Part model, mm, in its own coordinate system. Give positions to 0.01 mm unless a question says otherwise; leave off trailing zeros. Use a Markdown table: item, result. Add a question column.
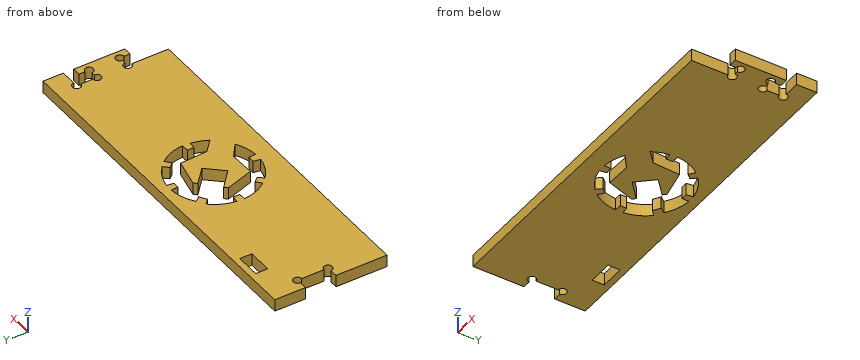
from build123d import *

# Parameters (mm, degrees)
SKETCH1_W           = 164.9
SKETCH1_H           = 55
BOSS_EXTRUDE1_DEPTH = 5.9
SKETCH2_W           = 5.9
SKETCH2_H           = 15
CUT_EXTRUDE1_DEPTH  = 6.9
BOSS_EXTRUDE2_DEPTH = 5.9
CUT_EXTRUDE2_DEPTH  = 10
SKETCH5_W           = 10
SKETCH5_H           = 10
BOSS_EXTRUDE3_DEPTH = 5.9
CUT_EXTRUDE3_REACH  = 7.9
SKETCH6_R           = 2.05
CUT_EXTRUDE4_REACH  = 7.9
SKETCH7_W           = 12
SKETCH7_H           = 5.9


with BuildPart() as part:
    # Sketch1 → Boss-Extrude1 (new body)
    with BuildSketch(Plane.XY):
        Rectangle(SKETCH1_W, SKETCH1_H)
    extrude(amount=BOSS_EXTRUDE1_DEPTH)

    # Sketch2 → Cut-Extrude1 (cut, through all)
    with BuildSketch(Plane.XY.offset(5.9)):
        with Locations((-79.5, 5)):
            Rectangle(SKETCH2_W, SKETCH2_H)
    extrude(amount=-CUT_EXTRUDE1_DEPTH, mode=Mode.SUBTRACT)

    # Sketch3 → Boss-Extrude2 (add)
    with BuildSketch(Plane.XY.offset(5.9)):
        Polygon((82.45, -7.5), (88.35, -7.5), (88.35, -12.5), (92.35, -12.5), (92.35, 12.5), (88.35, 12.5), (88.35, 7.5), (82.45, 7.5), align=None)
    extrude(amount=-BOSS_EXTRUDE2_DEPTH)

    # Sketch4 → Cut-Extrude2 (cut)
    with BuildSketch(Plane.XY.offset(5.9)):
        with BuildLine():
            Line((3.51583171, -15.706229716), (3.692822505, -19.080784973))
            ThreePointArc((3.692822505, -19.080784973), (9.080825588, -18.035079597), (14.033003188, -15.668644733))
            Line((14.033003188, -15.668644733), (7.525249631, -10.707966449))
            Line((7.525249631, -10.707966449), (-4.667323255, -11.041732232))
            Line((-4.667323255, -11.041732232), (-9.056316648, 2.465721032))
            Line((-9.056316648, 2.465721032), (-7.672540361, 3.987452797))
            Line((-7.672540361, 3.987452797), (0.63828327, -3.480150804))
            Line((0.63828327, -3.480150804), (7.889093057, 4.589420993))
            Line((7.889093057, 4.589420993), (0.219729645, 11.480963368))
            Line((0.219729645, 11.480963368), (1.603052795, 13.017301391))
            Line((1.603052795, 13.017301391), (15.495445969, 10.065059871))
            Line((15.495445969, 10.065059871), (16.237659976, -3.337384453))
            Line((16.237659976, -3.337384453), (21.895941701, -8.451220184))
            ThreePointArc((21.895941701, -8.451220184), (23.579573726, -4.648525456), (24.507536721, -0.594639829))
            Line((24.507536721, -0.594639829), (21.171770806, -0.180639971))
            ThreePointArc((21.171770806, -0.180639971), (21.286498935, 1.378538101), (21.285888417, 2.941931343))
            Line((21.285888417, 2.941931343), (24.837258291, 3.128195824))
            ThreePointArc((24.837258291, 3.128195824), (23.536690781, 9.458573353), (20.269548114, 15.034497878))
            Line((20.269548114, 15.034497878), (17.535016414, 12.941488009))
            ThreePointArc((17.535016414, 12.941488009), (16.508769514, 14.081533134), (15.445096221, 15.186741129))
            Line((15.445096221, 15.186741129), (17.692052457, 17.680150482))
            ThreePointArc((17.692052457, 17.680150482), (12.304554027, 21.210935864), (6.104308905, 22.956944215))
            Line((6.104308905, 22.956944215), (5.70284553, 19.6211861))
            ThreePointArc((5.70284553, 19.6211861), (4.176993745, 19.749298528), (2.645876068, 19.73154678))
            Line((2.645876068, 19.73154678), (2.474568352, 23.105152619))
            ThreePointArc((2.474568352, 23.105152619), (-3.819532601, 21.764454936), (-9.443176471, 18.635907879))
            Line((-9.443176471, 18.635907879), (-7.36611055, 15.97938168))
            ThreePointArc((-7.36611055, 15.97938168), (-9.138032671, 15.057329352), (-10.764172697, 13.897347837))
            Line((-10.764172697, 13.897347837), (-13.255215364, 16.14691078))
            ThreePointArc((-13.255215364, 16.14691078), (-16.804652941, 10.7695067), (-18.541993583, 4.564941506))
            Line((-18.541993583, 4.564941506), (-15.203305308, 4.160483172))
            ThreePointArc((-15.203305308, 4.160483172), (-15.337848427, 2.624728095), (-15.310082988, 1.083340867))
            Line((-15.310082988, 1.083340867), (-18.663730537, 0.907446652))
            ThreePointArc((-18.663730537, 0.907446652), (-17.372056658, -5.384049821), (-14.221680713, -10.981056224))
            Line((-14.221680713, -10.981056224), (-11.574159014, -8.917273625))
            ThreePointArc((-11.574159014, -8.917273625), (-10.549530454, -10.048759249), (-9.495391581, -11.15280392))
            Line((-9.495391581, -11.15280392), (-11.74257315, -13.641863724))
            ThreePointArc((-11.74257315, -13.641863724), (-6.357210629, -17.182483384), (-0.156549988, -18.940301546))
            Line((-0.156549988, -18.940301546), (0.271448667, -15.602569205))
            ThreePointArc((0.271448667, -15.602569205), (1.891578011, -15.718941802), (3.51583171, -15.706229716))
        make_face()
    extrude(amount=-CUT_EXTRUDE2_DEPTH, mode=Mode.SUBTRACT)

    # Sketch5 → Boss-Extrude3 (add)
    with BuildSketch(Plane(origin=(0, 0, 0), x_dir=(-1, 0, 0), z_dir=(0, 0, -1))):
        with Locations((-87.45, 22.5)):
            Rectangle(SKETCH5_W, SKETCH5_H)
    extrude(amount=-BOSS_EXTRUDE3_DEPTH)

    # Sketch6 → Cut-Extrude3 (cut, up to next)
    with BuildSketch(Plane(origin=(0, 0, 0), x_dir=(-1, 0, 0), z_dir=(0, 0, -1)), mode=Mode.PRIVATE) as cut_extrude3_sk1:
        with Locations((-82.45, -7.5)):
            Circle(SKETCH6_R)
    cut_extrude3_tool1 = extrude(cut_extrude3_sk1.sketch, amount=-CUT_EXTRUDE3_REACH, mode=Mode.PRIVATE) & part.part
    add(cut_extrude3_tool1.solids().sort_by_distance((82.45, -7.5, 0))[0], mode=Mode.SUBTRACT)
    # Sketch6 → Cut-Extrude3 (cut, up to next)
    with BuildSketch(Plane(origin=(0, 0, 0), x_dir=(-1, 0, 0), z_dir=(0, 0, -1)), mode=Mode.PRIVATE) as cut_extrude3_sk2:
        with Locations((-88.35, -7.5)):
            Circle(SKETCH6_R)
    cut_extrude3_tool2 = extrude(cut_extrude3_sk2.sketch, amount=-CUT_EXTRUDE3_REACH, mode=Mode.PRIVATE) & part.part
    add(cut_extrude3_tool2.solids().sort_by_distance((88.35, -7.5, 0))[0], mode=Mode.SUBTRACT)
    # Sketch6 → Cut-Extrude3 (cut, up to next)
    with BuildSketch(Plane(origin=(0, 0, 0), x_dir=(-1, 0, 0), z_dir=(0, 0, -1)), mode=Mode.PRIVATE) as cut_extrude3_sk3:
        with Locations((-88.35, 7.5)):
            Circle(SKETCH6_R)
    cut_extrude3_tool3 = extrude(cut_extrude3_sk3.sketch, amount=-CUT_EXTRUDE3_REACH, mode=Mode.PRIVATE) & part.part
    add(cut_extrude3_tool3.solids().sort_by_distance((88.35, 7.5, 0))[0], mode=Mode.SUBTRACT)
    # Sketch6 → Cut-Extrude3 (cut, up to next)
    with BuildSketch(Plane(origin=(0, 0, 0), x_dir=(-1, 0, 0), z_dir=(0, 0, -1)), mode=Mode.PRIVATE) as cut_extrude3_sk4:
        with Locations((-82.45, 7.5)):
            Circle(SKETCH6_R)
    cut_extrude3_tool4 = extrude(cut_extrude3_sk4.sketch, amount=-CUT_EXTRUDE3_REACH, mode=Mode.PRIVATE) & part.part
    add(cut_extrude3_tool4.solids().sort_by_distance((82.45, 7.5, 0))[0], mode=Mode.SUBTRACT)
    # Sketch6 → Cut-Extrude3 (cut, up to next)
    with BuildSketch(Plane(origin=(0, 0, 0), x_dir=(-1, 0, 0), z_dir=(0, 0, -1)), mode=Mode.PRIVATE) as cut_extrude3_sk5:
        with Locations((-82.45, 17.5)):
            Circle(SKETCH6_R)
    cut_extrude3_tool5 = extrude(cut_extrude3_sk5.sketch, amount=-CUT_EXTRUDE3_REACH, mode=Mode.PRIVATE) & part.part
    add(cut_extrude3_tool5.solids().sort_by_distance((82.45, 17.5, 0))[0], mode=Mode.SUBTRACT)
    # Sketch6 → Cut-Extrude3 (cut, up to next)
    with BuildSketch(Plane(origin=(0, 0, 0), x_dir=(-1, 0, 0), z_dir=(0, 0, -1)), mode=Mode.PRIVATE) as cut_extrude3_sk6:
        with Locations((76.55, 12.5)):
            Circle(SKETCH6_R)
    cut_extrude3_tool6 = extrude(cut_extrude3_sk6.sketch, amount=-CUT_EXTRUDE3_REACH, mode=Mode.PRIVATE) & part.part
    add(cut_extrude3_tool6.solids().sort_by_distance((-76.55, 12.5, 0))[0], mode=Mode.SUBTRACT)
    # Sketch6 → Cut-Extrude3 (cut, up to next)
    with BuildSketch(Plane(origin=(0, 0, 0), x_dir=(-1, 0, 0), z_dir=(0, 0, -1)), mode=Mode.PRIVATE) as cut_extrude3_sk7:
        with Locations((76.55, -2.5)):
            Circle(SKETCH6_R)
    cut_extrude3_tool7 = extrude(cut_extrude3_sk7.sketch, amount=-CUT_EXTRUDE3_REACH, mode=Mode.PRIVATE) & part.part
    add(cut_extrude3_tool7.solids().sort_by_distance((-76.55, -2.5, 0))[0], mode=Mode.SUBTRACT)

    # Sketch7 → Cut-Extrude4 (cut, up to next)
    with BuildSketch(Plane(origin=(0, 0, 0), x_dir=(-1, 0, 0), z_dir=(0, 0, -1)), mode=Mode.PRIVATE) as cut_extrude4_sk1:
        with Locations((57.45, 21.55)):
            Rectangle(SKETCH7_W, SKETCH7_H)
    cut_extrude4_tool1 = extrude(cut_extrude4_sk1.sketch, amount=-CUT_EXTRUDE4_REACH, mode=Mode.PRIVATE) & part.part
    add(cut_extrude4_tool1.solids().sort_by_distance((-57.45, 21.55, 0))[0], mode=Mode.SUBTRACT)


solid = part.part
1. Cut at A-A (z = 2). State how many separate pieces and enclosed holes the cut face has, plus the area to 3 significant figures.
2. Drill centre lines: probe 1 along Y at (x, z) = (-3, 3.2); probe 2 along X at (y, z) = (13.5, 1.15); probe 3 along X at (y, z) = (-14.5, 4.95). Where is each one in solid material? Low to high. Write a range as [from, to].
3. Pin check, flat tips, straight feed: P1, Ø8, axis at x = 11, y = 15, coming from the -Z side; P2, Ø2.5, axis at x = 82.45, y = -7.5, coming from the +Z side; P3, Ø1, axis at y = 5, z = 3.5, coming from the -X side; P4, Ø3, axis at y = 2.5, z = 4, coming from the +X side. Stop position of each tip, or through.
Responses:
| question | item | result |
|---|---|---|
| 1 | separate pieces | 1 |
| 1 | enclosed holes | 2 |
| 1 | area | 8,210 mm² |
| 2 | probe 1 | y = [-27.5, -18.39], [-11, -0.21], [22.05, 27.5] |
| 2 | probe 2 | x = [-82.45, -78.34], [-74.76, -15.3], [17.04, 18.26], [21.42, 82.45] |
| 2 | probe 3 | x = [-82.45, -10.73], [12.5, 82.45] |
| 3 | P1 | stops at z = 0 |
| 3 | P2 | passes through |
| 3 | P3 | stops at x = -76.55 |
| 3 | P4 | stops at x = 92.35 |
